Job drawing, mm, ordinate dimensions from the low corner. One solid piece. Round coordinates to 2 decimals unless told otherwise and drop trailing zeros. Loops run counter-clockwise (first coordinate to the right, second up) from the corner with the lowest first, then second, coordinate; pieces in that order, holes last. Notation, with made-up numbers: (6.25, 33.25) - (54.25, 33.25) arc R24 cw to (54.25, 61.25) - close; hole circle Ø8 at (40, 74). An arc over 180 degrees is marked (long way). Answer as CSV lines item,"result". Start each with the question number.
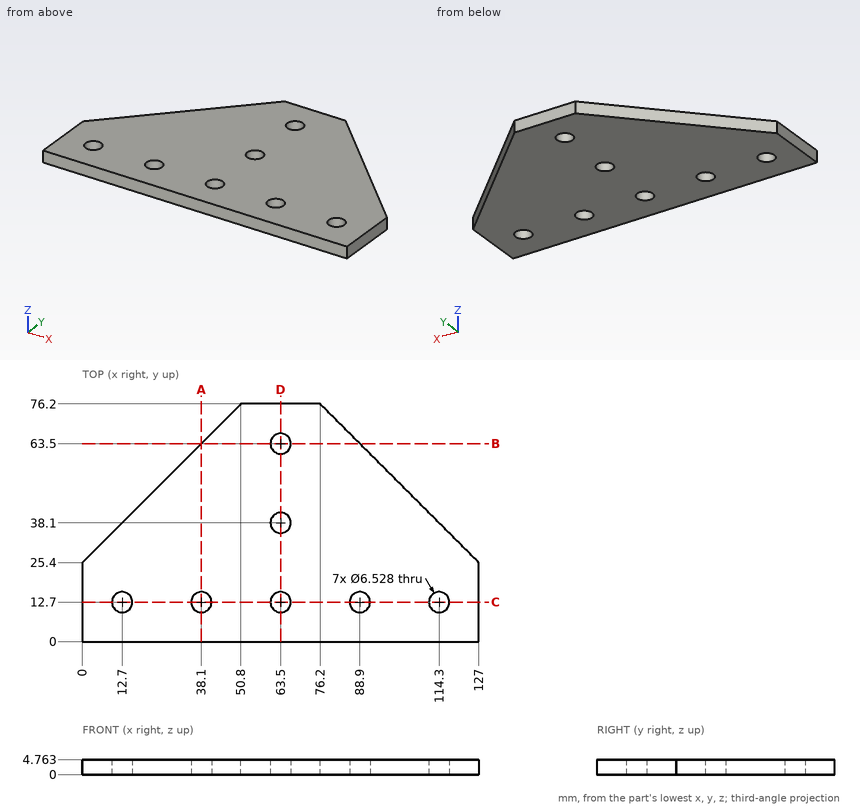
Q1. Band-saw the part on C-C, the plane y = 12.7. List the corners of the cut face in (x, z).
Q2. Band-saw the part on A-A, the plane x = 38.1. List the corners of the cut face in (y, z).
Q3. Wall check: probe 1 along Y at (x, z) = (63.5, 1.55); probe 2 along X at (y, z) = (12.7, 2.6); probe 3 along Y at (x, z) = (66.5, 3) (1 decimal). Give the ranges that are in metal, low to high. Write a range as [from, to].
Q4. Pin check, flat tips, straight feed: pin 1 Ø5 at (x, y) = (63.5, 63.5) entering from -Z; pin 2 Ø1.5 at (x, z) = (78, 0.5) entering from +Y. Stop position of each tip, or through.
Q5. Band-saw the part on D-D, the plane x = 63.5. List the corners of the cut face in (y, z).
Q6. Band-saw the part on B-B, the plane y = 63.5. List the corners of the cut face in (x, z).
Reported:
1,outline,"(0, 0) - (9.44, 0) - (9.44, 4.76) - (0, 4.76) - close; (15.96, 0) - (34.84, 0) - (34.84, 4.76) - (15.96, 4.76) - close; (41.36, 0) - (60.24, 0) - (60.24, 4.76) - (41.36, 4.76) - close; (66.76, 0) - (85.64, 0) - (85.64, 4.76) - (66.76, 4.76) - close; (92.16, 0) - (111.04, 0) - (111.04, 4.76) - (92.16, 4.76) - close; (117.56, 0) - (127, 0) - (127, 4.76) - (117.56, 4.76) - close"
2,outline,"(0, 0) - (9.44, 0) - (9.44, 4.76) - (0, 4.76) - close; (15.96, 0) - (63.5, 0) - (63.5, 4.76) - (15.96, 4.76) - close"
3,probe 1,"y = [0, 9.44], [15.96, 34.84], [41.36, 60.24], [66.76, 76.2]"
3,probe 2,"x = [0, 9.44], [15.96, 34.84], [41.36, 60.24], [66.76, 85.64], [92.16, 111.04], [117.56, 127]"
3,probe 3,"y = [0, 11.4], [14, 36.8], [39.4, 62.2], [64.8, 76.2]"
4,pin 1,"passes through"
4,pin 2,"stops at y = 75.15"
5,outline,"(0, 0) - (9.44, 0) - (9.44, 4.76) - (0, 4.76) - close; (15.96, 0) - (34.84, 0) - (34.84, 4.76) - (15.96, 4.76) - close; (41.36, 0) - (60.24, 0) - (60.24, 4.76) - (41.36, 4.76) - close; (66.76, 0) - (76.2, 0) - (76.2, 4.76) - (66.76, 4.76) - close"
6,outline,"(38.1, 0) - (60.24, 0) - (60.24, 4.76) - (38.1, 4.76) - close; (66.76, 0) - (88.9, 0) - (88.9, 4.76) - (66.76, 4.76) - close"
